Autodesk Inventor part; units mm, degrees
ref_plane "YZ Plane" through (0, 0, 0) normal (1, 0, 0) x (0, 1, 0)
ref_plane "XZ Plane" through (0, 0, 0) normal (0, 1, 0) x (-1, 0, 0)
ref_plane "XY Plane" through (0, 0, 0) normal (0, 0, 1) x (1, 0, 0)
sketch "Sketch1" plane through (0, 0, 0) normal (0, 1, 0) x (-1, 0, 0)
  line L0 (0, 0) -> (0, -3)
  line L1 (-250, -38) -> (-250, -78)
  line L2 (0, 0) -> (-20, 0)
  line L3 (-50, 0) -> (-50, -3)
  line L4 (-50, 0) -> (-70, 0)
  line L5 (-70, 0) -> (-70, -3)
  line L6 (-100, 0) -> (-100, -3)
  line L7 (-100, 0) -> (-120, 0)
  line L8 (-120, 0) -> (-120, -3)
  line L9 (-150, 0) -> (-150, -3)
  line L10 (-150, 0) -> (-170, 0)
  line L11 (-170, 0) -> (-170, -3)
  line L12 (-200, 0) -> (-200, -3)
  line L13 (-200, 0) -> (-220, 0)
  line L14 (-220, 0) -> (-220, -3)
  line L15 (-20, 0) -> (-20, -3)
  line L16 (-250, -58) -> (-250, -78)
  line L17 (-250, -78) -> (-247, -78)
  line L18 (-247, -78) -> (-247, -113)
  line L19 (-250, -58) -> (-250, -38)
  line L20 (-250, -38) -> (-247, -38)
  line L21 (-247, -38) -> (-247, -3)
  line L22 (-220, -3) -> (-247, -3)
  line L23 (-170, -3) -> (-200, -3)
  line L24 (-120, -3) -> (-150, -3)
  line L25 (-20, -3) -> (-50, -3)
  line L26 (-70, -3) -> (-100, -3)
  line L27 (0, -116) -> (0, -113)
  line L28 (0, -116) -> (-20, -116)
  line L29 (-50, -116) -> (-50, -113)
  line L30 (-50, -116) -> (-70, -116)
  line L31 (-70, -116) -> (-70, -113)
  line L32 (-100, -116) -> (-100, -113)
  line L33 (-100, -116) -> (-120, -116)
  line L34 (-120, -116) -> (-120, -113)
  line L35 (-150, -116) -> (-150, -113)
  line L36 (-150, -116) -> (-170, -116)
  line L37 (-170, -116) -> (-170, -113)
  line L38 (-200, -116) -> (-200, -113)
  line L39 (-200, -116) -> (-220, -116)
  line L40 (-220, -116) -> (-220, -113)
  line L41 (-20, -116) -> (-20, -113)
  line L42 (-3, -58) -> (-3, -78)
  line L43 (-3, -78) -> (0, -78)
  line L44 (-3, -58) -> (-3, -38)
  line L45 (-3, -38) -> (0, -38)
  line L46 (0, -113) -> (0, -78)
  line L47 (0, -38) -> (0, -3)
  line L48 (-50, -113) -> (-20, -113)
  line L49 (-100, -113) -> (-70, -113)
  line L50 (-150, -113) -> (-120, -113)
  line L51 (-247, -113) -> (-220, -113)
  line L52 (-200, -113) -> (-170, -113)
  line L53 (-20, -53) -> (-20, -56)
  line L54 (-20, -56) -> (-45, -56)
  line L55 (-45, -56) -> (-45, -53)
  line L56 (-113, -53) -> (-113, -56)
  line L57 (-113, -56) -> (-88, -56)
  line L58 (-88, -56) -> (-88, -53)
  line L59 (-20, -53) -> (-45, -53)
  line L60 (-88, -53) -> (-113, -53)
  line L61 (-63, -51) -> (-66.9, -51)
  line L62 (-66.9, -51) -> (-66.9, -47.1)
  line L63 (-66.9, -47.1) -> (-59.1, -47.1)
  line L64 (-59.1, -47.1) -> (-59.1, -51)
  line L65 (-59.1, -51) -> (-63, -51)
  circle A0 centre (-88, -46.5) radius 4.5
  line L66 (-37, -49.5) -> (-28, -49.5)
  line L67 (-28, -49.5) -> (-28, -38.5)
  line L68 (-28, -38.5) -> (-37, -38.5)
  line L69 (-37, -38.5) -> (-37, -49.5)
  line L70 (-32.5, -38.5) -> (-32.5, -38)
  line L71 (-32.5, -34.5) -> (-26.7, -34.5)
  line L72 (-26.7, -34.5) -> (-26.7, -30.5)
  line L73 (-26.7, -30.5) -> (-38.3, -30.5)
  line L74 (-38.3, -30.5) -> (-38.3, -34.5)
  line L75 (-38.3, -34.5) -> (-32.5, -34.5)
  dimension "d2" = 110
  dimension "d3" = 20
  dimension "d4" = 20
  dimension "d5" = 20
  dimension "d7" = 20
  dimension "d8" = 20
  dimension "d9" = 20
  dimension "d10" = 3
  dimension "d11" = 20
  dimension "d12" = 3
  dimension "d13" = 250
  dimension "d14" = 30
  dimension "d15" = 30
  dimension "d16" = 30
  dimension "d17" = 30
  dimension "d25" = 25
  dimension "d26" = 25
  dimension "d27" = 17
  dimension "d29" = 110
  dimension "d30" = 43
  dimension "d31" = 57
  dimension "d32" = 3
  dimension "d37" = 3.9
  dimension "d38" = 7.8
  dimension "d39" = 60
  dimension "d40" = 2
  dimension "d44" = 9
  dimension "d46" = 78
  dimension "d47" = 3
  dimension "d48" = 6.5
  dimension "d49" = 3
  dimension "d50" = 3
  dimension "d51" = 11
  dimension "d52" = 53
  dimension "d53" = 2
  dimension "d55" = 3.5
  dimension "d57" = 8
  dimension "d58" = 25
  dimension "d60" = 4
  dimension "d62" = 4
  dimension "d63" = 11.6
  dimension "d64" = 9
extrude "Extrusion3" add sketch "Sketch1" along normal blind 3
properties part number "latPort"
Check sheet for the modelled part. Datum: model origin and axes. Units: mm. Round coordinates to 2 decimals unless told otherwise and drop trailing zeros. Loops run counter-clockwise (first coordinate to the right, second up) from the corner with the lowest first, then second, coordinate; pieces in that order, holes last. Notation, with made-up numbers: M 53,82 L 95,82 A28 ccw 95,107 Z; hole C 5.5,4.5 d2. An arc over 180 degrees is marked long. One line per question, with ' | ' between items. Start each with the question number.
Item 1: Gauge pin test, flat ends, axial feed: pin 1 Ø1.5 at (x, y) = (248, 2) entering from +Z; pin 2 Ø1.5 at (x, y) = (129.5, 2) entering from -Z. Record the tip position at first contact, or that the pin passes through.
Item 2: Section check A-A (x = 77). Record the boundary of the cut face in (y, z).
Item 3: Release check for a two-part mould opening along Z. For faces 1 (the face through (91.6, 1.5, -43.8)), 2 (the face through (127, 0, -57)) record: released by +Z, released by -Z, zero draft, split by the parting line, or undercut.
Item 4: Section check B-B (y = 1.75). State how many separate pieces and enclosed holes the cut face has, and give its area (3 significant figures).
Item 5: Scan lines: probe 1 along Z at (x, y) = (35.5, 2.85); probe 2 along X at (y, z) = (1.8, -31); probe 3 along X at (y, z) = (0.4, -87). Record each from-to range of solid material in increasing order.
Worked out:
1) pin 1: z = -38 | pin 2: z = -113
2) outline: M 0,-113 L 3,-113 L 3,-3 L 0,-3 Z
3) face 1: undercut | face 2: zero draft
4) separate pieces: 1 | enclosed holes: 6 | area: 27,400 mm^2
5) probe 1: -113 to -56, -53 to -49.5, -38.5 to -34.5, -30.5 to -3 | probe 2: 0 to 26.7, 38.3 to 247 | probe 3: 0 to 247
